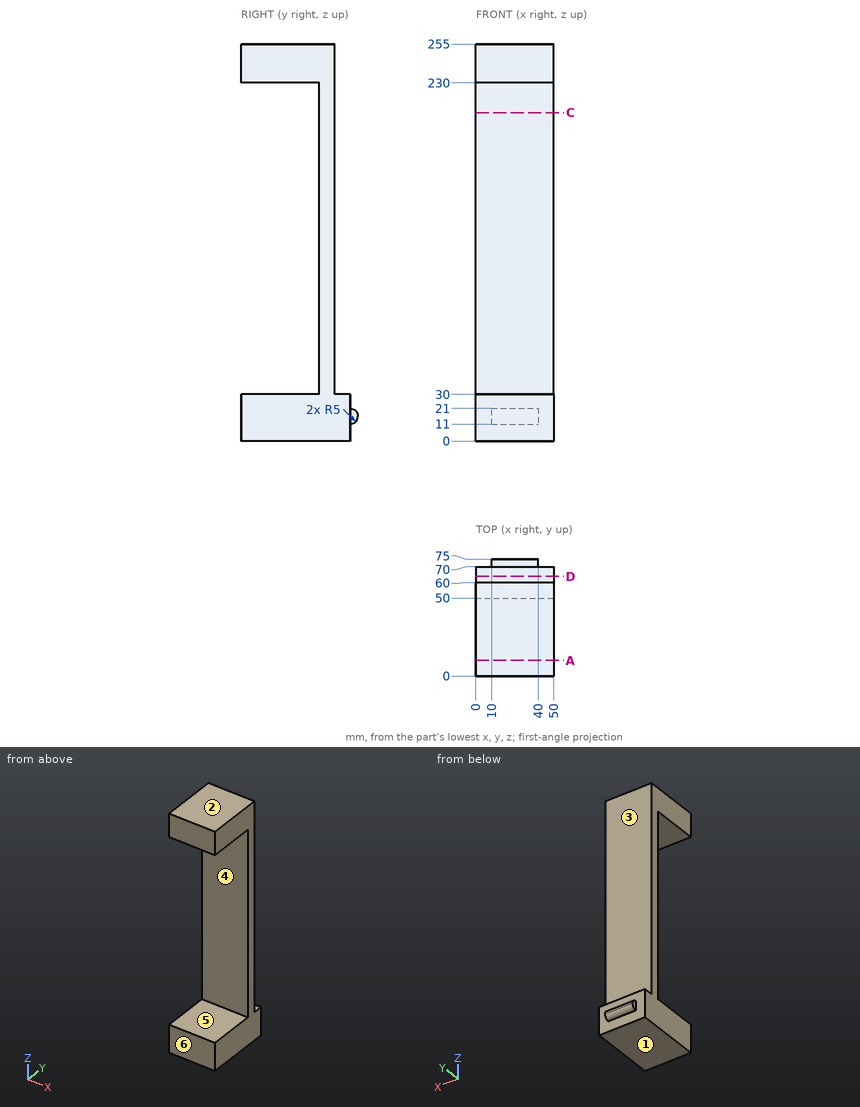
Study the drawing (mm; zero at the part's minimum x, y, z) and answer. A direction names the side the tool comes from. Give positions to 0.01 mm unless a question says otherwise; leave off trailing zeros. Loops run counter-clockwise (first coordinate to the right, second up) from the corner with the lowest first, then second, coordinate; pieces in that order, holes last. Notation, with made-up numbers: (-33, -18.75) -> (-28, -18.75) arc R15 ccw to (-28, -9.75) -> close; hole circle Ø9 at (23.25, 29). An arc over 180 degrees is marked (long way). Write item = value, one per line. Start each with the question number.
(1) Find section D-D on y = 64. Give the vertices of the cut face in (x, z), and give its area (3 significant figures).
(2) Find section A-A on y = 10. Give the vertices of the cut face in (x, z), and give its area (3 significant figures).
(3) Which of the six approach directions +Z, -Z, +X, -X, +Y, -Y give full straight-line access (tool end or side, diameter ignored) to the marked faces 5 and 6?
(4) Find section C-C on z = 211. Give the vertices of the cut face in (x, y).
(5) Given pin 1 Ø1.5 at (y, z) = (73.5, 18) entering from -X; pin 2 Ø5.5 at (y, z) = (73.5, 14) entering from +X; pin 3 Ø15 at (x, z) = (25, 127) entering from +Y, each flat-ended and moving along its own axis, determine where each tip first touches the part or whether it passes through.
(6) The mould has two halves that part along Z. Classify the marked faces 1, 2, 3 and 4: +Z half, -Z half, draft (parallel to the pull), parting line (faces both ways), or undercut.
(7) Find the intervals of material crossed by probe 1 along Z at (x, y) = (28, 4); probe 2 along Y at (x, z) = (48.5, 152.5); probe 3 along Z at (x, y) = (11, 67.5), in increasing order. Write a range as from..to.
From the geometry:
q1.outline = (0, 0) -> (50, 0) -> (50, 30) -> (0, 30) -> close
q1.area = 1,500 mm^2
q2.outline = (0, 0) -> (50, 0) -> (50, 30) -> (0, 30) -> close; (0, 230) -> (50, 230) -> (50, 255) -> (0, 255) -> close
q2.area = 2,750 mm^2
q3.face_5 = +X, -X, -Y
q3.face_6 = +Z, -Z, +X, -X, -Y
q4.outline = (0, 50) -> (50, 50) -> (50, 60) -> (0, 60) -> close
q5.pin_1 = 10
q5.pin_2 = 40
q5.pin_3 = 60
q6.face_1 = -Z half
q6.face_2 = +Z half
q6.face_3 = draft
q6.face_4 = undercut
q7.probe_1 = 0..30, 230..255
q7.probe_2 = 50..60
q7.probe_3 = 0..30
